Input: dimensioned drawing with shaded views. Units: mm. Origin: part minimum x, y, z. Round coordinates to 2 decimals unless told otherwise and drop trailing zeros. Loops run counter-clockwise (first coordinate to the right, second up) from the corner with the lowest first, then second, coordinate; pieces in that order, holes last. Notation, with made-up numbers: (33, 26.25) - (77, 26.25) arc R20 cw to (77, 32.25) - close; hole circle Ø10 at (6.25, 72.25). An arc over 180 degrees is marked (long way). One line per question, with ' | ' between items.
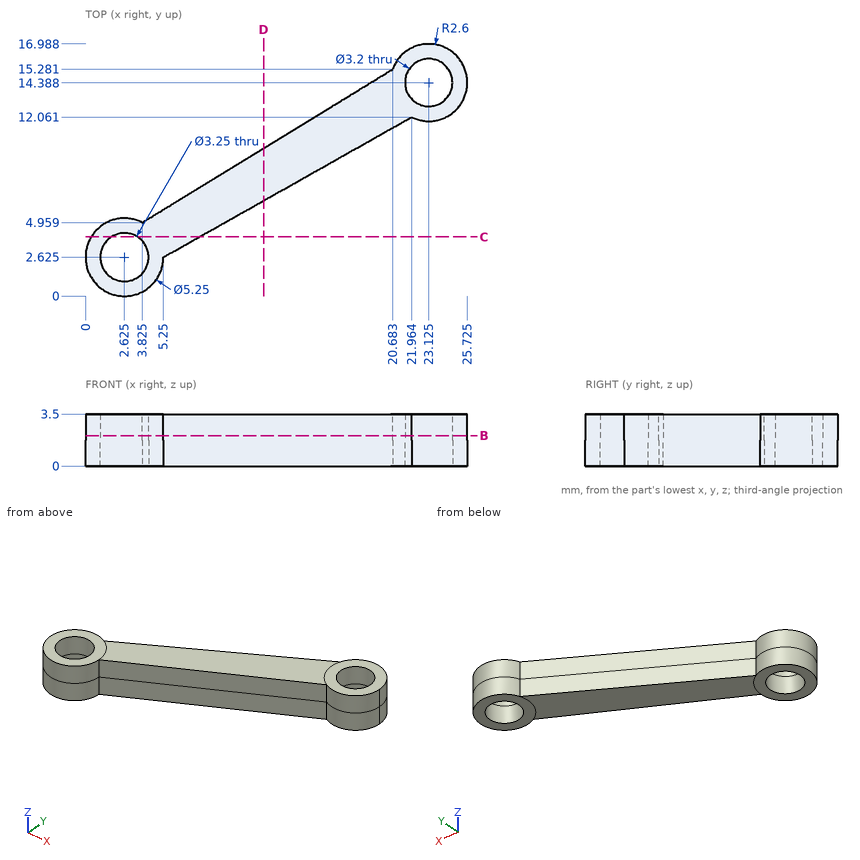
1. Section query B-B, the plane z = 2.05. Give the number of separate pieces and of enclosed holes in the cut face.
Worked out:
separate pieces: 1 | enclosed holes: 2
2. Section query C-C, the plane y = 4. Return loops of the section in (x, z) (1 decimal), plus the area to 3 significant figures.
Worked out:
outline: (0.4, 0) - (1.8, 0) - (1.8, 3.5) - (0.4, 3.5) - close; (3.5, 0) - (7.7, 0) - (7.7, 3.5) - (3.5, 3.5) - close | area: 19.5 mm2
3. Material intervals for probe 1 along Y at (x, z) = (23, 2.75) (1 decimal); probe 2 along Y at (x, z) = (24.5, 2.75) (1 decimal); probe 3 along X at (y, z) = (13, 0.3) (1 decimal), sorted ascending.
Worked out:
probe 1: y = 11.8 to 12.8, 16 to 17 | probe 2: y = 12.2 to 13.6, 15.2 to 16.6 | probe 3: x = 17 to 22.3, 23.9 to 25.3
4. Contact query for flat-ended pins moving along their axis: P1, Ø3.5, axis at x = 23.12, y = 14.39, coming from the +Z side; P2, Ø1.5, axis at x = 6.5, z = 0.5, coming from the -Y side; P3, Ø2, axis at x = 6.5, z = 1, coming from the +Y side; P4, Ø1.5, axis at y = 14, z = 2.5, coming from the -X side (1 decimal). Output: stop coordinate, or through.
Worked out:
P1: stops at z = 3.5 | P2: stops at y = 2.91 | P3: stops at y = 7.21 | P4: stops at x = 17.4
5. Section query D-D, the plane x = 12. Return loops of the section in (y, z) (1 decimal).
Worked out:
outline: (6.4, 0) - (10, 0) - (10, 3.5) - (6.4, 3.5) - close
